The figure shows three views and two pictorial views of one solid part (mm, origin at its lowest corner). Answer the questions. A direction names the side the tool comes from. Round coordinates to 2 decimals unless told otherwise and drop trailing zeros. Write each loop counter-clockwise with the first axis right and the second up, starting at its lowest first coordinate (ties: lowest second). Pieces come first, ordered by that corner, then holes. Notation, with made-up numbers: M 1.5,34.25 L 37.5,34.25 A30 ccw 37.5,66.25 Z; hole C -16,6 d10. An arc over 180 degrees is marked long. One line per item, written item: value. Start each with the question number.
Q1. Find section B-B (z = 17). Write down the section's boundary in (x, y) (3 decimals), and give its area (3 significant figures).
Q2. The mould has two halves that part along Y. Classify the marked faces 1, 2 and 3: released by +Y, released by -Y, zero draft, split by the parting line, or undercut.
Q3. A tool of negligible diameter and unlimited length cuts with its end or side. For the marked faces 4 and 5, from which of +Z, -Z, +X, -X, +Y, -Y can it reach the whole face along a straight path? Write none if from no direction.
Q4. Consider probe 1 along Y at (x, z) = (39.37, 16.35) (3 decimals); probe 2 along Y at (x, z) = (39.37, 5.75); probe 3 along X at (y, z) = (39, 14). Determine where each line is inside the solid, lowest interval first.
Q5. Find section C-C (x = 71.12). Write down the section's boundary in (y, z) (1 decimal), and give its area (3 significant figures).
Q6. Given pin 1 Ø8.5 at (x, y) = (37.5, 32.5) entering from -Z (3 decimals); pin 2 Ø4 at (x, y) = (39.37, 7.62) entering from +Z; pin 3 Ø1.5 at (x, z) = (34, 4.5) entering from -Y; pin 4 Ø8 at (x, y) = (39.37, 39.37) entering from -Z (3 decimals), each flat-ended and moving along its own axis, determine where each tip first touches the part or whether it passes through.
Q7. Find section A-A (x = 39.37). Count the separate pieces of the cut face and the enclosed holes in it.
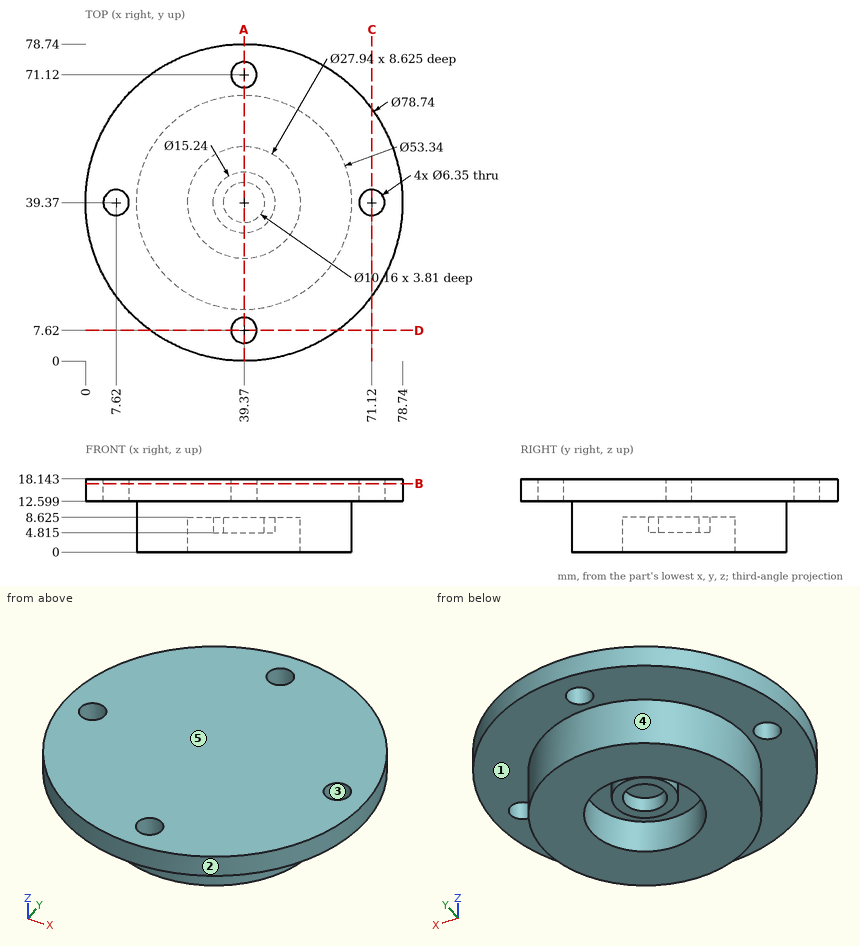
The answers:
1. outline: C 39.37,39.37 d78.74; hole C 7.62,39.37 d6.35; hole C 39.37,7.62 d6.35; hole C 39.37,71.12 d6.35; hole C 71.12,39.37 d6.35
1. area: 4,740 mm2
2. face 1: zero draft
2. face 2: split by the parting line
2. face 3: undercut
3. face 4: -Z
3. face 5: +Z, +X, -X, +Y, -Y
4. probe 1: 0 to 4.445, 10.795 to 67.945, 74.295 to 78.74
4. probe 2: 12.7 to 25.4, 31.75 to 34.29, 44.45 to 46.99, 53.34 to 66.04
4. probe 3: 0 to 4.47, 10.77 to 67.97, 74.27 to 78.74
5. outline: M 16.1,12.6 L 36.2,12.6 L 36.2,18.1 L 16.1,18.1 Z; M 42.5,12.6 L 62.6,12.6 L 62.6,18.1 L 42.5,18.1 Z
5. area: 223 mm2
6. pin 1: z = 4.815
6. pin 2: through
6. pin 3: y = 13.1
6. pin 4: z = 8.625
7. separate pieces: 3
7. enclosed holes: 0
